Check sheet for the modelled part. Datum: model origin and axes. Units: mm. Round coordinates to 2 decimals unless told otherwise and drop trailing zeros. Loops run counter-clockwise (first coordinate to the right, second up) from the corner with the lowest first, then second, coordinate; pieces in that order, holes last. Notation, with made-up numbers: (30, 29.5) -> (70, 29.5) arc R15 cw to (70, 52.5) -> close; hole circle Ø7 at (84.25, 74). An arc over 180 degrees is marked (long way). Return JSON: item names as keys, results as strings.
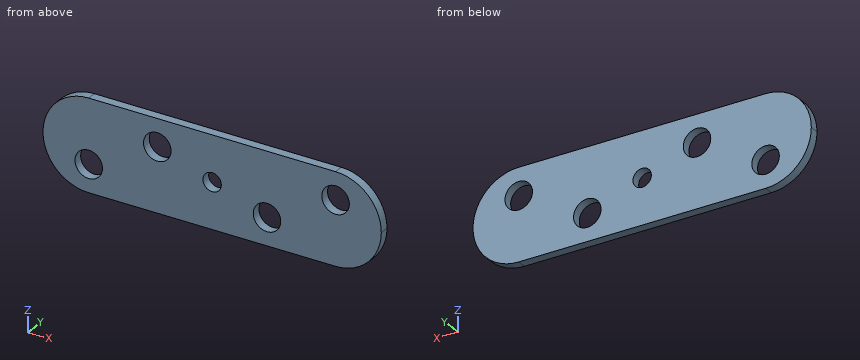
from build123d import *

# Parameters (mm, degrees)
F1_DEPTH = 2
F3_D     = 6.02
F5_D     = 4.02


with BuildPart() as f1:
    # F0 (on Front) → F1 (new body)
    with BuildSketch(Plane.XZ):
        with BuildLine():
            ThreePointArc((37, 0), (34.071068, 7.071068), (27, 10))
            Line((27, 10), (-27, 10))
            ThreePointArc((-27, 10), (-34.071068, 7.071068), (-37, 0))
            ThreePointArc((-37, 0), (-34.071068, -7.071068), (-27, -10))
            Line((-27, -10), (27, -10))
            ThreePointArc((27, -10), (34.071068, -7.071068), (37, 0))
        make_face()
    extrude(amount=F1_DEPTH)

    # F3 (through all)
    with Locations(Plane.XZ.offset(2)):
        with Locations((-12, 4), (-27, -4), (27, 4), (12, -4)):
            Hole(F3_D / 2)

    # F5 (through all)
    with Locations(Plane.XZ.offset(2)):
        with Locations((0, 0)):
            Hole(F5_D / 2)


solid = f1.part
Q1. Section check D-D (x = 0). Record the boundary of the cut face in (y, z), then the cut area to 3 significant figures.
Results list:
{"outline": "(-2, -10) -> (0, -10) -> (0, -2.01) -> (-2, -2.01) -> close; (-2, 2.01) -> (0, 2.01) -> (0, 10) -> (-2, 10) -> close", "area": "32.0 mm^2"}
Q2. Go/stop test with a flat-tipped pin: pin 1 (3.5 mm diameter, centred on x = -27, z = -4, fed in from +Y). Record where the tip stops, or that it passes through.
Results list:
{"pin 1": "through"}
Q3. Section check C-C (z = 6.25). Record the boundary of the cut face in (x, y), then the cut area to 3 significant figures.
Results list:
{"outline": "(-34.81, -2) -> (-14, -2) -> (-14, 0) -> (-34.81, 0) -> close; (-10, -2) -> (25, -2) -> (25, 0) -> (-10, 0) -> close; (29, -2) -> (34.81, -2) -> (34.81, 0) -> (29, 0) -> close", "area": "123 mm^2"}
Q4. Section check B-B (y = -1). Record the boundary of the cut face in (x, z).
Results list:
{"outline": "(-37, 0) arc R10 ccw to (-27, -10) -> (27, -10) arc R10 ccw to (37, 0) arc R10 ccw to (27, 10) -> (-27, 10) arc R10 ccw to start; hole circle Ø6.02 at (-27, -4); hole circle Ø6.02 at (-12, 4); hole circle Ø4.02 at (0, 0); hole circle Ø6.02 at (12, -4); hole circle Ø6.02 at (27, 4)"}
Q5. Material ranges on line 1 (Z direction, x = 12, y = -0.4); line 2 (Z direction, x = 27, y = -1); line 3 (X direction, y = -0.55, z = 2.5), recorded low to high.
Results list:
{"line 1": "-10 to -7.01, -0.99 to 10", "line 2": "-10 to 0.99, 7.01 to 10", "line 3": "-36.68 to -14.61, -9.39 to 24.39, 29.61 to 36.68"}
Q6. Section check A-A (x = 12). Record the boundary of the cut face in (y, z).
Results list:
{"outline": "(-2, -10) -> (0, -10) -> (0, -7.01) -> (-2, -7.01) -> close; (-2, -0.99) -> (0, -0.99) -> (0, 10) -> (-2, 10) -> close"}
